The drawing under review shows one solid part. Ordinate dimensions are in mm from its lowest x, y, z. A direction names the side the tool comes from. Coordinates: 2 decimals unless noted, no trailing zeros. Loops run counter-clockwise (first coordinate to the right, second up) from the corner with the lowest first, then second, coordinate; pieces in that order, holes last. Notation, with made-up numbers: (-4.5, 25.5) - (19.5, 25.5) arc R32 ccw to (19.5, 58.5) - close; hole circle Ø9 at (-29.75, 38). An arc over 180 degrees is marked (long way). Answer as a JSON object with one key per item and string values. Group by question number.
Item 1: Mouldability with a two-part tool opening along Z and no side actions: class the marked faces 4, 5 and 6 as released by +Z, released by -Z, zero draft, split by the parting line, or undercut.
Item 2: To check wall thickness, follow line 1 (Y direction, x = 37.5, z = 70.75); line 2 (Z direction, x = 37.5, y = 22); line 3 (X direction, y = 21, z = 37) (3 decimals). State the ranges of each line that lie inside material, in increasing order.
Item 3: We need section C-C (x = 37.5). Give the boundary of the cut face in (y, z), then the cut area to 4 significant figures.
Item 4: We need section B-B (z = 37.5). Give the boundary of the cut face in (x, y).
Item 5: Tool access review of the marked faces 1, 2 and 3: name each direction out of +Z, -Z, +X, -X, +Y, -Y from which nothing blocks a thin tool from reaching the whole face with its end or side.
Item 6: We need section A-A (y = 7.5). Give the boundary of the cut face in (x, z).
Item 7: We need section D-D (x = 60.5). Give the boundary of the cut face in (y, z), then the cut area to 3 significant figures.
Item 8: Clearance check with flat-ended pins moving along their axes: pin 1 (3 mm diameter, centred on x = 65.5, y = 6.5, fed in from +Z); pin 2 (6 mm diameter, centred on x = 63, y = 6, fed in from +Z); pin 3 (12.5 mm diameter, centred on x = 5.5, z = 31.5, fed in from -Y); pin 4 (10 mm diameter, centred on x = 24, z = 52, fed in from +Y). State where each tip first meets the part, or that it passes through.
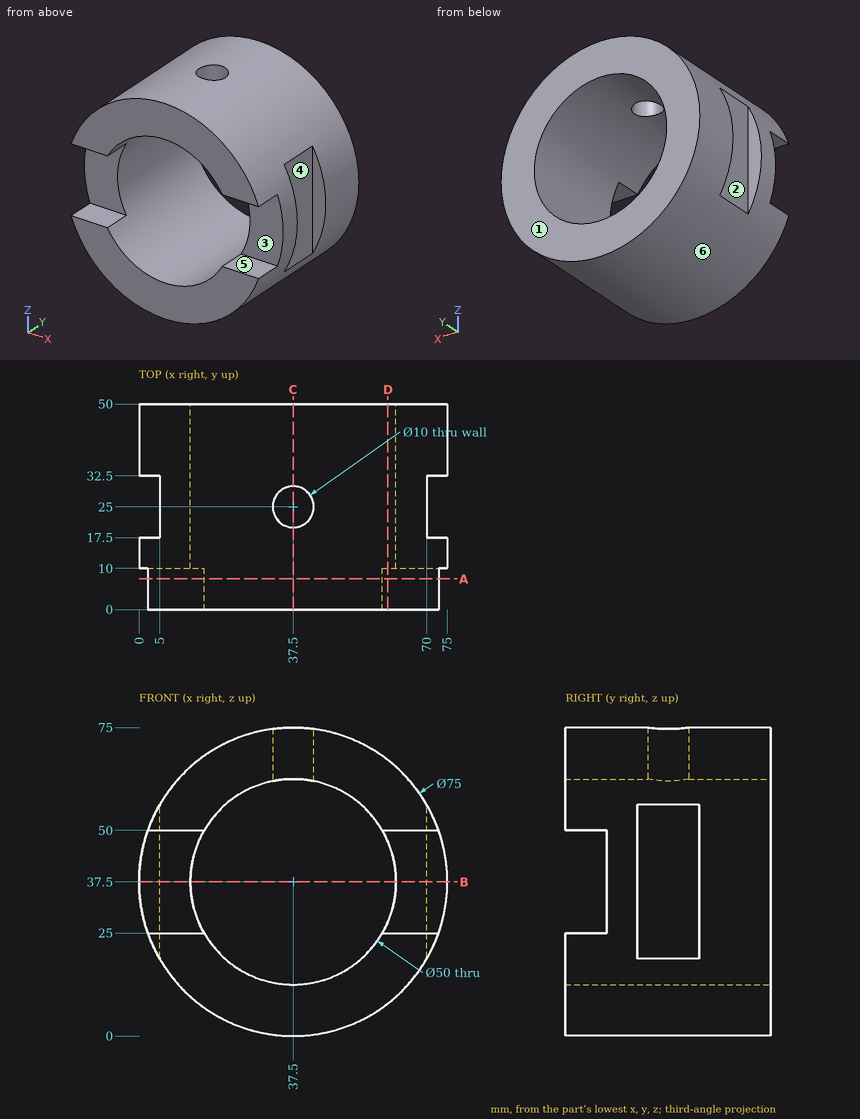
Check sheet entries:
{
 "1": {"face 4": "zero draft", "face 5": "undercut", "face 6": "split by the parting line"},
 "2": {"line 1": "y = 0 to 20, 30 to 50", "line 2": "z = 0 to 12.5", "line 3": "x = 5 to 12.505, 62.495 to 70"},
 "3": {"outline": "(0, 0) - (50, 0) - (50, 12.5) - (0, 12.5) - close; (0, 62.5) - (20, 62.5) - (20, 75) - (0, 75) - close; (30, 62.5) - (50, 62.5) - (50, 75) - (30, 75) - close", "area": "1,125 mm2"},
 "4": {"outline": "(0, 10) - (12.5, 10) - (12.5, 50) - (0, 50) - (0, 32.5) - (5, 32.5) - (5, 17.5) - (0, 17.5) - close; (62.5, 10) - (75, 10) - (75, 17.5) - (70, 17.5) - (70, 32.5) - (75, 32.5) - (75, 50) - (62.5, 50) - close"},
 "5": {"face 1": "+Z, -Z, +X, -X, +Y", "face 2": "+Z, -Z, -X", "face 3": "+X, -X, -Y"},
 "6": {"outline": "(2.14, 25) arc R37.5 ccw to (72.86, 25) - (59.15, 25) arc R25 cw to (15.85, 25) - close; (2.14, 50) - (15.85, 50) arc R25 cw to (59.15, 50) - (72.86, 50) arc R37.5 ccw to start"},
 "7": {"outline": "(0, 7.88) - (50, 7.88) - (50, 27.7) - (10, 27.7) - (10, 25) - (0, 25) - close; (0, 50) - (10, 50) - (10, 47.3) - (50, 47.3) - (50, 67.12) - (0, 67.12) - close", "area": "1,930 mm2"},
 "8": {"pin 1": "stops at z = 64.03", "pin 2": "stops at z = 67.5", "pin 3": "stops at y = 10", "pin 4": "passes through"}
}
